Can you work these out from the model? Positions are in its coordinate system, mm. A direction names the side the tool comes from. Give positions to 0.01 mm unless a question says otherwise; leave off trailing zeros. Write each loop counter-clockwise with the first axis right and the second up, starting at its lowest first coordinate (ties: lowest second). Pieces come first, ordered by that corner, then holes.
1. Suppose I cut it at A-A (x = 62). Please give me the cut outline in (y, z).
2. Thinking about a two-plate mould opening in X: for faces 1 (the flat face through (316.203, 28.694, 0.022)), 2 (the flat face through (42.337, 376.449, 0.022)), 3 (the cylindrical face through (139.011, -126.566, 0.022)), which applies, pulls with the +X half, pulls with the -X half, needs draft (parallel to the pull), parting line crosses it, or undercut?
3. Suppose I cut it at C-C (y = 110). Please give me the cut outline in (x, z).
4. I'm going to push flat-ended pins straight in: pin 1 (1.5 mm diameter, centred on y = 306, z = -0.5, fed in from +X); pin 2 (1 mm diameter, centred on x = 301, z = 0, fed in from +Y); pin 3 (1 mm diameter, centred on y = -40, z = 0, fed in from -X). Where does each tip first touch, or does it pass through?
5. If I drill on probe 1 along Y at (x, z) = (264, 1); probe 2 along Y at (x, z) = (82, -0.85); probe 3 along Y at (x, z) = (210.5, -0.75), over which ranges is the centre line in solid material (lowest first)?
6. On a 3-axis mill with a long thin cutter (end or side, diameter ignored), from which of +Z, -Z, +X, -X, +Y, -Y can I reach the whole of each face in a straight line? I mean faces 4 (the flat face through (207.5, -284.8, 0)), 5 (the cylindrical face through (85.544, -468.765, 0.022)). Say none if no direction works.
7. Suppose I cut it at B-B (z = 0.15). Give the number of separate pieces and of enclosed holes in the cut face, and give its area (3 significant figures).
```python
from build123d import *

# Parameters (mm, degrees)
SKETCH1_R          = 6.35
BASE_EXTRUDE_DEPTH = 1.5875
SKETCH4_R          = 9.525
CUT_EXTRUDE1_DEPTH = 632.57042153


with BuildPart() as part:
    # Sketch1 → Base-Extrude (new, symmetric)
    with BuildSketch(Plane.XY):
        with BuildLine():
            Line((1.016, 288.028470779), (1.016, 152.396613296))
            ThreePointArc((1.016, 152.396613296), (108.121687001, 107.40326252), (152.4, 0))
            Line((152.4, 0), (224.08509271, 0))
            ThreePointArc((224.08509271, 0), (226.970303426, 8.05977117), (234.315000004, 12.45747334))
            Line((234.315000004, 12.45747334), (400.41570649, 45.392253319))
            ThreePointArc((400.41570649, 45.392253319), (416.586287434, 56.182910854), (420.390467759, 75.247385412))
            Line((420.390467759, 75.247385412), (408.040004229, 137.534752113))
            ThreePointArc((408.040004229, 137.534752113), (397.249346694, 153.705333057), (378.184872136, 157.509513382))
            Line((378.184872136, 157.509513382), (224.103045939, 126.957861002))
            ThreePointArc((224.103045939, 126.957861002), (209.958830275, 134.414849048), (214.319609154, 149.79825293))
            Line((214.319609154, 149.79825293), (343.449482538, 240.752562825))
            ThreePointArc((343.449482538, 240.752562825), (353.849089047, 257.177366098), (349.588631557, 276.145088156))
            Line((349.588631557, 276.145088156), (313.021911166, 328.059681094))
            ThreePointArc((313.021911166, 328.059681094), (296.597107893, 338.459287603), (277.629385835, 334.198830112))
            Line((277.629385835, 334.198830112), (135.364166743, 233.992468211))
            ThreePointArc((135.364166743, 233.992468211), (120.264827781, 234.342028255), (116.177210875, 248.881753745))
            Line((116.177210875, 248.881753745), (178.82248253, 413.942798461))
            ThreePointArc((178.82248253, 413.942798461), (178.240047031, 433.374389929), (164.087992844, 446.702755935))
            Line((164.087992844, 446.702755935), (104.719933894, 469.234590669))
            ThreePointArc((104.719933894, 469.234590669), (85.288342425, 468.65215517), (71.95997642, 454.500100983))
            Line((71.95997642, 454.500100983), (11.87361179, 296.181398599))
            ThreePointArc((11.87361179, 296.181398599), (7.625816745, 290.532130708), (1.016, 288.028470779))
        make_face()
        with Locations((395.475521078, 70.3072)):
            Circle(SKETCH1_R, mode=Mode.SUBTRACT)
        with Locations((383.125057548, 132.594566701)):
            Circle(SKETCH1_R, mode=Mode.SUBTRACT)
        with Locations((328.822794382, 261.5184)):
            Circle(SKETCH1_R, mode=Mode.SUBTRACT)
        with Locations((292.256073991, 313.432992937)):
            Circle(SKETCH1_R, mode=Mode.SUBTRACT)
        with Locations((155.07525895, 422.955532355)):
            Circle(SKETCH1_R, mode=Mode.SUBTRACT)
        with Locations((95.7072, 445.487367089)):
            Circle(SKETCH1_R, mode=Mode.SUBTRACT)
    base_extrude = extrude(amount=BASE_EXTRUDE_DEPTH, both=True)

    # Sketch4 → Cut-Extrude1 (cut, through all)
    with BuildSketch(Plane.XY.offset(1.5875)):
        with Locations((181.882606251, 28.80868)):
            Circle(SKETCH4_R)
        with Locations((164.07826617, 83.603499153)):
            Circle(SKETCH4_R)
        with Locations((130.212802196, 130.214625308)):
            Circle(SKETCH4_R)
        with Locations((83.601201897, 164.07943668)):
            Circle(SKETCH4_R)
        with Locations((28.806133473, 181.883009581)):
            Circle(SKETCH4_R)
    cut_extrude1 = extrude(amount=-CUT_EXTRUDE1_DEPTH, mode=Mode.SUBTRACT)

    # Mirror1: Base-Extrude, Cut-Extrude1 across plane
    add(base_extrude.mirror(Plane.ZX))
    add(cut_extrude1.mirror(Plane.ZX), mode=Mode.SUBTRACT)


solid = part.part
```
Checks:
1. outline: (-428.26, -1.59) - (-139.22, -1.59) - (-139.22, 1.59) - (-428.26, 1.59) - close; (139.22, -1.59) - (428.26, -1.59) - (428.26, 1.59) - (139.22, 1.59) - close
2. face 1: pulls with the +X half
2. face 2: pulls with the -X half
2. face 3: undercut
3. outline: (105.48, -1.59) - (413.5, -1.59) - (413.5, 1.59) - (105.48, 1.59) - close
4. pin 1: stops at x = 329.09
4. pin 2: stops at y = 337.46
4. pin 3: stops at x = 146.92
5. probe 1: y = -324.6 to -184.79, -134.87 to -18.34, 18.34 to 134.87, 184.79 to 324.6
5. probe 2: y = -466.87 to -173.47, -154.69 to -128.46, 128.46 to 154.69, 173.47 to 466.87
5. probe 3: y = -286.92 to -145.53, -133.3 to 133.3, 145.53 to 286.92
6. face 4: +Z, -Z
6. face 5: +Z, -Z, -Y
7. separate pieces: 1
7. enclosed holes: 22
7. area: 196,000 mm2
